The listing builds one solid part. Answer for the finished solid, in the listing's coordinates (mm). Face numbers are marked on the shaded views. A direction names the side the tool comes from. Give positions to 0.01 mm unless a question says otherwise; leave off trailing zeros. Order: outer loops, then holes, each group sorted by start corner. A loop starts at its lowest first (then second) coordinate and runs counter-clockwise, first axis right, second up. Notation, with made-up numbers: (-35, 50) -> (24, 50) arc R20 ccw to (24, 63) -> close; hole circle Ø6 at (77.5, -11.5). An arc over 180 degrees is marked (long way). Answer as a JSON object with one key per item and string values. Group by question number.
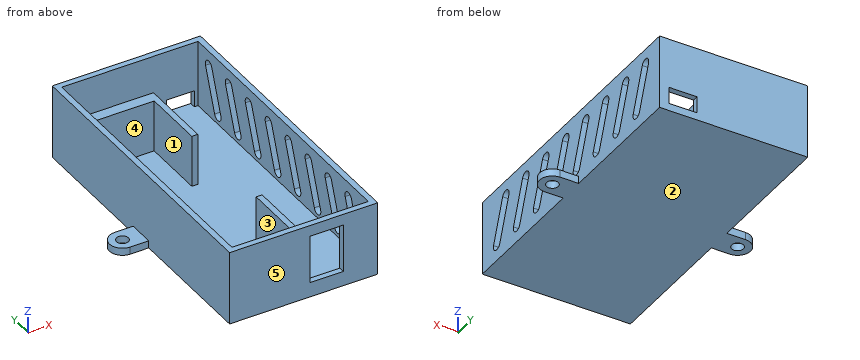
```python
from build123d import *

# Parameters (mm, degrees)
F1_DEPTH  = 20
F2_DEPTH  = 2
F0_W      = 1.6
F0_H      = 20
F3_DEPTH  = 16
F4_W      = 9
F4_H      = 13
F5_DEPTH  = 10
F7_DEPTH  = 5
F8_W      = 7.5
F8_H      = 4.5
F9_DEPTH  = 5
F0_R      = 1.6
F10_DEPTH = 2


with BuildPart() as f1:
    # F0 (on Top) → F1 (new body)
    with BuildSketch(Plane.XY):
        Polygon((-40, 0), (0, 0), (0, 36.5), (0, 43.5), (0, 80), (-40, 80), (-40, 43.5), (-40, 36.5), align=None)
        Polygon((-1.6, 78.4), (-1.6, 1.6), (-18.3, 1.6), (-19.9, 1.6), (-38.4, 1.6), (-38.4, 67.6), (-38.4, 70.6), (-38.4, 78.4), align=None, mode=Mode.SUBTRACT)
    extrude(amount=F1_DEPTH)

    # F0 (on Top) → F2 (join)
    with BuildSketch(Plane.XY):
        Polygon((-18.3, 1.6), (-1.6, 1.6), (-1.6, 78.4), (-38.4, 78.4), (-38.4, 70.6), (-18.3, 70.6), (-18.3, 50.6), (-19.9, 50.6), (-19.9, 67.6), (-38.4, 67.6), (-38.4, 1.6), (-19.9, 1.6), (-19.9, 21.6), (-18.3, 21.6), align=None)
    extrude(amount=F2_DEPTH)

    # F0 (on Top) → F3 (join)
    with BuildSketch(Plane.XY):
        Polygon((-18.3, 70.6), (-38.4, 70.6), (-38.4, 67.6), (-19.9, 67.6), (-19.9, 50.6), (-18.3, 50.6), align=None)
        with Locations((-19.1, 11.6)):
            Rectangle(F0_W, F0_H)
    extrude(amount=F3_DEPTH)

    # F4 (on face) → F5 (cut)
    with BuildSketch(Plane.XZ):
        with Locations((-13.8, 10.5)):
            Rectangle(F4_W, F4_H)
    extrude(amount=-F5_DEPTH, mode=Mode.SUBTRACT)

    # F6 (on face) → F7 (cut)
    with BuildSketch(Plane.YZ):
        with BuildLine():
            Line((9.194703, 16.289342), (5.090461, 5.01303))
            ThreePointArc((5.090461, 5.01303), (5.98697, 3.090461), (7.909539, 3.98697))
            Line((7.909539, 3.98697), (12.013781, 15.263281))
            ThreePointArc((12.013781, 15.263281), (11.117272, 17.18585), (9.194703, 16.289342))
        make_face()
        with BuildLine():
            Line((16.909539, 3.98697), (21.013781, 15.263281))
            ThreePointArc((21.013781, 15.263281), (20.117272, 17.18585), (18.194703, 16.289342))
            Line((18.194703, 16.289342), (14.090461, 5.01303))
            ThreePointArc((14.090461, 5.01303), (14.98697, 3.090461), (16.909539, 3.98697))
        make_face()
        with BuildLine():
            Line((25.909539, 3.98697), (30.013781, 15.263281))
            ThreePointArc((30.013781, 15.263281), (29.117272, 17.18585), (27.194703, 16.289342))
            Line((27.194703, 16.289342), (23.090461, 5.01303))
            ThreePointArc((23.090461, 5.01303), (23.98697, 3.090461), (25.909539, 3.98697))
        make_face()
        with BuildLine():
            Line((34.909539, 3.98697), (39.013781, 15.263281))
            ThreePointArc((39.013781, 15.263281), (38.117272, 17.18585), (36.194703, 16.289342))
            Line((36.194703, 16.289342), (32.090461, 5.01303))
            ThreePointArc((32.090461, 5.01303), (32.98697, 3.090461), (34.909539, 3.98697))
        make_face()
        with BuildLine():
            Line((43.909539, 3.98697), (48.013781, 15.263281))
            ThreePointArc((48.013781, 15.263281), (47.117272, 17.18585), (45.194703, 16.289342))
            Line((45.194703, 16.289342), (41.090461, 5.01303))
            ThreePointArc((41.090461, 5.01303), (41.98697, 3.090461), (43.909539, 3.98697))
        make_face()
        with BuildLine():
            Line((52.909539, 3.98697), (57.013781, 15.263281))
            ThreePointArc((57.013781, 15.263281), (56.117272, 17.18585), (54.194703, 16.289342))
            Line((54.194703, 16.289342), (50.090461, 5.01303))
            ThreePointArc((50.090461, 5.01303), (50.98697, 3.090461), (52.909539, 3.98697))
        make_face()
        with BuildLine():
            Line((61.909539, 3.98697), (66.013781, 15.263281))
            ThreePointArc((66.013781, 15.263281), (65.117272, 17.18585), (63.194703, 16.289342))
            Line((63.194703, 16.289342), (59.090461, 5.01303))
            ThreePointArc((59.090461, 5.01303), (59.98697, 3.090461), (61.909539, 3.98697))
        make_face()
        with BuildLine():
            Line((70.909539, 3.98697), (75.013781, 15.263281))
            ThreePointArc((75.013781, 15.263281), (74.117272, 17.18585), (72.194703, 16.289342))
            Line((72.194703, 16.289342), (68.090461, 5.01303))
            ThreePointArc((68.090461, 5.01303), (68.98697, 3.090461), (70.909539, 3.98697))
        make_face()
    extrude(amount=-F7_DEPTH, mode=Mode.SUBTRACT)

    # F8 (on face) → F9 (cut)
    with BuildSketch(Plane(origin=(0, 80, 0), x_dir=(-1, 0, 0), z_dir=(0, 1, 0))):
        with Locations((6.35, 4.25)):
            Rectangle(F8_W, F8_H)
    extrude(amount=-F9_DEPTH, mode=Mode.SUBTRACT)

    # F0 (on Top) → F10 (join)
    with BuildSketch(Plane.XY):
        with BuildLine():
            Line((-45, 36.5), (-40, 36.5))
            Line((-40, 36.5), (-40, 43.5))
            Line((-40, 43.5), (-45, 43.5))
            ThreePointArc((-45, 43.5), (-48.5, 40), (-45, 36.5))
        make_face()
        with Locations((-45, 40)):
            Circle(F0_R, mode=Mode.SUBTRACT)
        with BuildLine():
            Line((0, 43.5), (0, 36.5))
            Line((0, 36.5), (5, 36.5))
            ThreePointArc((5, 36.5), (8.5, 40), (5, 43.5))
            Line((5, 43.5), (0, 43.5))
        make_face()
        with Locations((5, 40)):
            Circle(F0_R, mode=Mode.SUBTRACT)
    extrude(amount=F10_DEPTH)


solid = f1.part
```
(1) A cutting plane is placed at A-A (x = -13.5). Determine the outline of the cut face in (y, z).
(2) A cutting plane is placed at B-B (y = 42.5). Determine the outline of the cut face in (x, z).
(3) Find the intervals of material crossed by line 1 along Y through (x, z) = (-30.5, 6.75); line 2 along Y through (x, z) = (-45, 0.65); line 3 along Y through (x, z) = (-25, 17.25), in increasing order. Write a range as [from, to].
(4) A cutting plane is placed at C-C (x = -22). Determine the outline of the cut face in (y, z).
(5) Which of the six approach directions +Z, -Z, +X, -X, +Y, -Y give full straight-line access (tool end or side, diameter ignored) to the marked faces 1 and 2?
(6) Flat-ended cylindrical pins translate along their axes: pin 1 Ø1.3 at (x, z) = (-19.5, 9.5) entering from -Y; pin 2 Ø1 at (x, z) = (2.5, 1.5) entering from -Y; pin 3 Ø3.5 at (x, y) = (-45, 40) entering from +Z; pin 4 Ø2 at (y, z) = (14.5, 13.5) entering from +X. Find the tip coordinate at first contact, or state that the pin passes through.
(7) For a pull along X with two mould halves and no side action, classify the marked faces 3, 4 and 5 as +X half, -X half, draft (parallel to the pull), parting line (faces both ways), or undercut.
(8) A cutting plane is placed at D-D (y = 15.5). Determine the outline of the cut face in (x, z), and give its area (3 significant figures).
Check sheet entries:
{
 "1": {"outline": "(0, 0) -> (80, 0) -> (80, 20) -> (78.4, 20) -> (78.4, 2) -> (1.6, 2) -> (1.6, 4) -> (0, 4) -> close; (0, 17) -> (1.6, 17) -> (1.6, 20) -> (0, 20) -> close"},
 "2": {"outline": "(-47.45, 0) -> (7.45, 0) -> (7.45, 2) -> (0, 2) -> (0, 3) -> (-1.6, 3) -> (-1.6, 2) -> (-38.4, 2) -> (-38.4, 20) -> (-40, 20) -> (-40, 2) -> (-47.45, 2) -> close; (-1.6, 8.89) -> (0, 8.89) -> (0, 20) -> (-1.6, 20) -> close"},
 "3": {"line 1": "y = [0, 1.6], [67.6, 70.6], [78.4, 80]", "line 2": "y = [36.5, 38.4], [41.6, 43.5]", "line 3": "y = [0, 1.6], [78.4, 80]"},
 "4": {"outline": "(0, 0) -> (80, 0) -> (80, 20) -> (78.4, 20) -> (78.4, 2) -> (70.6, 2) -> (70.6, 16) -> (67.6, 16) -> (67.6, 2) -> (1.6, 2) -> (1.6, 20) -> (0, 20) -> close"},
 "5": {"face 1": "+Z", "face 2": "-Z, +X, -X, +Y, -Y"},
 "6": {"pin 1": "stops at y = 0", "pin 2": "stops at y = 36.5", "pin 3": "stops at z = 2", "pin 4": "stops at x = 0"},
 "7": {"face 3": "undercut", "face 4": "undercut", "face 5": "draft"},
 "8": {"outline": "(-40, 0) -> (0, 0) -> (0, 3) -> (-1.6, 3) -> (-1.6, 2) -> (-18.3, 2) -> (-18.3, 16) -> (-19.9, 16) -> (-19.9, 2) -> (-38.4, 2) -> (-38.4, 20) -> (-40, 20) -> close; (-1.6, 8.89) -> (0, 8.89) -> (0, 20) -> (-1.6, 20) -> close", "area": "151 mm2"}
}
